Answer from the drawing. Dimensions are ordinates in mm from the lowest x, y and z of the part. A direction names the side the tool comes from. Give positions to 0.01 mm unless a question says otherwise; leave off trailing zeros. Loops run counter-clockwise (first coordinate to the right, second up) from the corner with the lowest first, then second, coordinate; pieces in that order, holes last. Notation, with made-up numbers: (20, -26) - (36, -26) arc R14 cw to (36, -8) - close; hole circle Ø10 at (49.25, 32). An arc over 180 degrees is marked (long way). One line per question, with ' | ' between items. Start each with the question number.
1. For a pull along X with two mould halves and no side action, classify the marked faces 3, 4 and 5 as released by +X, released by -X, zero draft, split by the parting line, or undercut.
2. Section D-D (y = 26.5) is taken. Determine the outline of the cut face in (x, z).
3. Section C-C (x = 17) is taken. Determine the outline of the cut face in (y, z).
4. Section A-A (z = 6.35) is taken. Determine the outline of the cut face in (x, y), plus the area to 3 significant figures.
5. Section B-B (x = 6.35) is taken. Determine the outline of the cut face in (y, z).
6. Find the intervals of material crossed by line 1 (X direction, y = 2.25, z = 6.35); line 2 (Z direction, x = 6.35, y = 4.5); line 3 (Y direction, x = 11, z = 8.5), in increasing order.
7. Which of the six approach directions +Z, -Z, +X, -X, +Y, -Y give full straight-line access (tool end or side, diameter ignored) to the marked faces 1 and 2?
8. This flat-tipped pin is pushed along its axis until it touches: pin 1 (19 mm diameter, centred on x = 12, y = 26.5, fed in from -Z). Where does it stop, or does it pass through?
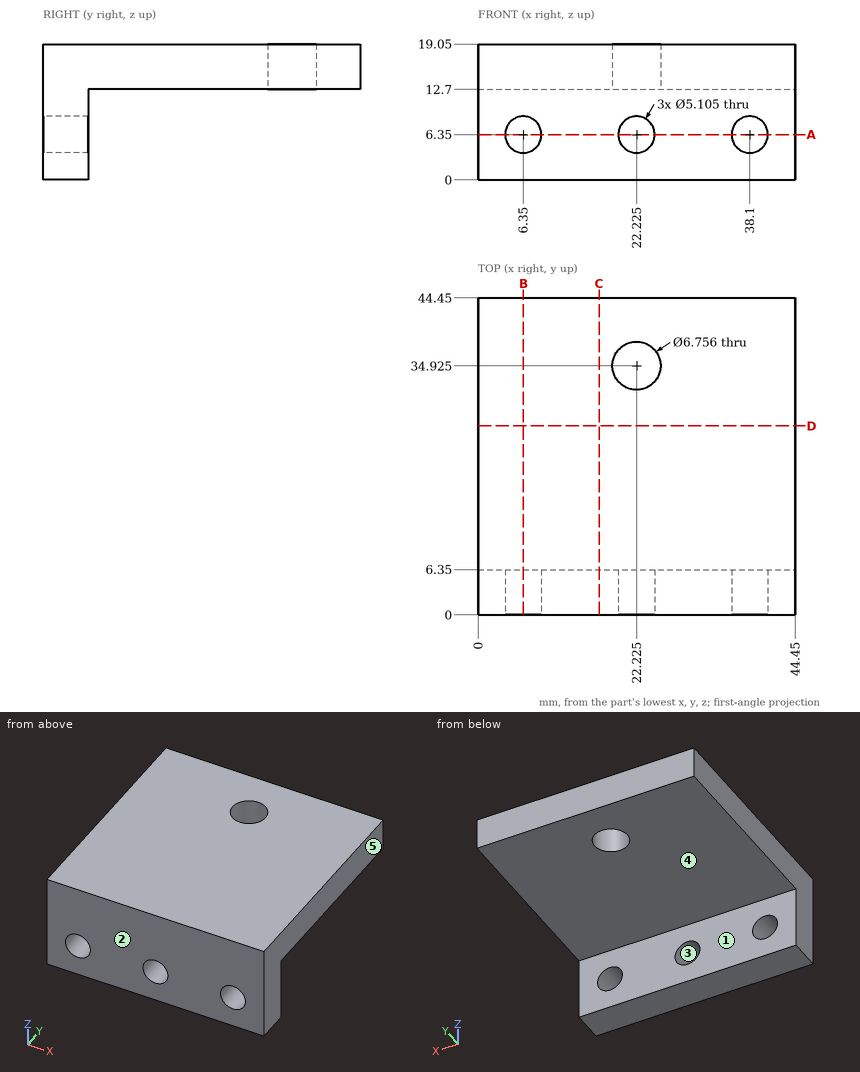
Conclusion:
1) face 3: undercut | face 4: zero draft | face 5: released by +X
2) outline: (0, 12.7) - (44.45, 12.7) - (44.45, 19.05) - (0, 19.05) - close
3) outline: (0, 0) - (6.35, 0) - (6.35, 12.7) - (44.45, 12.7) - (44.45, 19.05) - (0, 19.05) - close
4) outline: (0, 0) - (3.8, 0) - (3.8, 6.35) - (0, 6.35) - close; (8.9, 0) - (19.67, 0) - (19.67, 6.35) - (8.9, 6.35) - close; (24.78, 0) - (35.55, 0) - (35.55, 6.35) - (24.78, 6.35) - close; (40.65, 0) - (44.45, 0) - (44.45, 6.35) - (40.65, 6.35) - close | area: 185 mm²
5) outline: (0, 0) - (6.35, 0) - (6.35, 3.8) - (0, 3.8) - close; (0, 8.9) - (6.35, 8.9) - (6.35, 12.7) - (44.45, 12.7) - (44.45, 19.05) - (0, 19.05) - close
6) line 1: 0 to 3.8, 8.9 to 19.67, 24.78 to 35.55, 40.65 to 44.45 | line 2: 0 to 3.8, 8.9 to 19.05 | line 3: 0 to 6.35
7) face 1: -Z, +X, -X, +Y | face 2: +Z, -Z, +X, -X, -Y
8) pin 1: z = 12.7
